Could you check a few things on this model? Use its own coordinates, in mm. A direction names the side the tool comes from. Round coordinates to 2 decimals unless told otherwise and drop trailing zeros. Write each loop counter-clockwise with the first axis right and the second up, starting at its lowest first coordinate (ties: lowest second). Pieces come first, ordered by that corner, then holes. Notation, with made-up numbers: M 26.5,86.25 L 69.5,86.25 A23 ccw 69.5,100.25 Z; hole C -14,61 d11. An arc over 180 degrees is marked long. One line per item, written item: value. Start each with the question number.
(1) I'm going to push flat-ended pins straight in: pin 1 Ø1 at (x, y) = (-13, 1.5) entering from +Z; pin 2 Ø12 at (x, z) = (5.5, -12) entering from -Y; pin 3 Ø2 at (y, z) = (1, -5) entering from +X. Where does each tip first touch, or does it pass through?
(2) I want a section at A-A on x = 7. Please give me the cut outline in (y, z).
(3) I want a section at B-B on y = 0. Please give me the cut outline in (x, z), and give its area (3 significant figures).
(4) Which directions (+Z, -Z, +X, -X, +Y, -Y) give clear straight access to the entire face, cutting with the end or side of a thin tool? Please do faces 1 (the face through (58, 0, -20)), 2 (the face through (28, 0, -17)).
(5) If I drill on L1, parallel to Z at x = 28.5, y = -0.25; L2, parallel to Z at x = 5.5, y = 1.25; L3, parallel to Y at x = -3, z = -20, over which ranges is the centre line in solid material (lowest first)?
Autodesk Inventor part; units mm, degrees
ref_plane "YZ Plane" through (0, 0, 0) normal (1, 0, 0) x (0, 1, 0)
ref_plane "XZ Plane" through (0, 0, 0) normal (0, 1, 0) x (-1, 0, 0)
ref_plane "XY Plane" through (0, 0, 0) normal (0, 0, 1) x (1, 0, 0)
sketch "Esboço1" plane through (0, 0, 0) normal (1, 0, 0) x (0, 1, 0)
  line L0 (0, 0) -> (15, 0)
  circle A0 centre (0, -20) radius 3
revolve "Revolução1" add sketch "Esboço1" angle 180 about axis through (0, 0, 0) along (0, 1, 0)
sketch "Esboço2" plane through (0, 0, 20) normal (1, 0, 0) x (0, 0, -1)
  circle A0 centre (0, 0) radius 3
  circle A1 centre (40, 0) radius 3
  point P0 (20, 0)
extrude "Extrusão1" add sketch "Esboço2" along normal blind 58
chamfer "Chanfro1" distance 0.5 angle 45 2 edges at (58, 0, -17) (58, 0, 23)
sketch "Esboço3" plane through (0, 0, 0) normal (0, 1, 0) x (-1, 0, 0)
  point P0 (0, 0)
thread "Rosca1"
thread "Rosca2"
properties part number "parafuso u abraçadeira" material "Aço inoxidável"
Found:
1. pin 1: stops at z = 18.94
1. pin 2: stops at y = -2.24
1. pin 3: stops at x = -16
2. outline: C 0,-20 d6; C 0,20 d6
3. outline: M 0,-23 L 57.5,-23 L 58,-22.5 L 58,-17.5 L 57.5,-17 L 0,-17 A17 cw 0,17 L 57.5,17 L 58,17.5 L 58,22.5 L 57.5,23 L 0,23 A23 ccw Z
3. area: 1,070 mm²
4. face 1: +Z, -Z, +X, +Y, -Y
4. face 2: +X
5. L1: z = -22.99 to -17.01, 17.01 to 22.99
5. L2: z = -22.73 to -17.27, 17.27 to 22.73
5. L3: y = -2.99 to 2.99
